Autodesk Inventor part; units mm, degrees
ref_plane "YZ Plane" through (0, 0, 0) normal (1, 0, 0) x (0, 1, 0)
ref_plane "XZ Plane" through (0, 0, 0) normal (0, 1, 0) x (-1, 0, 0)
ref_plane "XY Plane" through (0, 0, 0) normal (0, 0, 1) x (1, 0, 0)
sketch "Sketch1" plane through (0, 0, 0) normal (0, 0, 1) x (1, 0, 0)
  arc A0 (2, 32) -> (0, 30) centre (2, 30) ccw
  line L0 (0, 30) -> (0, 20)
  line L1 (15, 20) -> (0, 20)
  line L2 (15, 30) -> (15, 20)
  arc A1 (15, 30) -> (13, 32) centre (13, 30) ccw
  line L3 (13, 32) -> (2, 32)
  arc A2 (0, -10) -> (2, -12) centre (2, -10) ccw
  line L4 (13, -12) -> (2, -12)
  arc A3 (13, -12) -> (15, -10) centre (13, -10) ccw
  line L5 (15, -10) -> (15, 0)
  line L6 (15, 0) -> (0, 0)
  line L7 (0, -10) -> (0, 0)
  line L8 (15, 20) -> (15, 0)
  line L9 (0, 20) -> (0, 0)
  point P0 (15, 24)
extrude "Extrusion1" add sketch "Sketch1" along normal blind 5
sketch "Sketch2" plane through (0, 0, 5) normal (0, 0, 1) x (1, 0, 0)
  circle A0 centre (7.5, -6) radius 1.2
  line L0 (15, -10) -> (15, 30)
  circle A1 centre (7.5, 26) radius 1.2
  point P0 (0, 0)
  dimension "d2" = 2.4
  dimension "d3" = 7.5
  dimension "d4" = 2.4
extrude "Extrusion2" cut sketch "Sketch2" against normal up to surface (5 mm away)
properties part number "ramie 03-3"
Read the model definition and answer for the solid it produces. Units are mm, in the model's axes. Round coordinates to 2 decimals unless told otherwise and drop trailing zeros. Write each loop counter-clockwise with the first axis right and the second up, starting at its lowest first coordinate (ties: lowest second). Pieces come first, ordered by that corner, then holes.
1. The part is cut by section C-C, the plane z = 2. Determine the outline of the cut face in (x, y), then the cut area to 3 significant figures.
2. The part is cut by section B-B, the plane x = 7.5. Determine the outline of the cut face in (y, z).
3. The part is cut by section A-A, the plane y = 26. Determine the outline of the cut face in (x, z).
4. Determine the mould class of faces 1 (the face through (7.24, 24.83, 2.54)), 2 (the face through (6.3, -5.95, 2.54)), 3 (the face through (14.43, -11.4, 2.46)), 4 (the face through (15, 10, 2)) for opening direction Y: pulls with the +Y half, pulls with the -Y half, needs draft (parallel to the pull), parting line crosses it, or undercut.
5. Straight lines are drawn through the part: L1, parallel to Y at x = 7.5, z = 2.15; L2, parallel to Y at x = 1.75, z = 0.3; L3, parallel to Y at x = 1.5, z = 1.3. For each, find the intervals that lie inside material, in ascending order.
Values:
1. outline: (0, -10) arc R2 ccw to (2, -12) - (13, -12) arc R2 ccw to (15, -10) - (15, 30) arc R2 ccw to (13, 32) - (2, 32) arc R2 ccw to (0, 30) - close; hole circle Ø2.4 at (7.5, -6); hole circle Ø2.4 at (7.5, 26)
1. area: 648 mm2
2. outline: (-12, 0) - (-7.2, 0) - (-7.2, 5) - (-12, 5) - close; (-4.8, 0) - (24.8, 0) - (24.8, 5) - (-4.8, 5) - close; (27.2, 0) - (32, 0) - (32, 5) - (27.2, 5) - close
3. outline: (0, 0) - (6.3, 0) - (6.3, 5) - (0, 5) - close; (8.7, 0) - (15, 0) - (15, 5) - (8.7, 5) - close
4. face 1: undercut
4. face 2: undercut
4. face 3: pulls with the -Y half
4. face 4: needs draft
5. L1: y = -12 to -7.2, -4.8 to 24.8, 27.2 to 32
5. L2: y = -11.98 to 31.98
5. L3: y = -11.94 to 31.94
